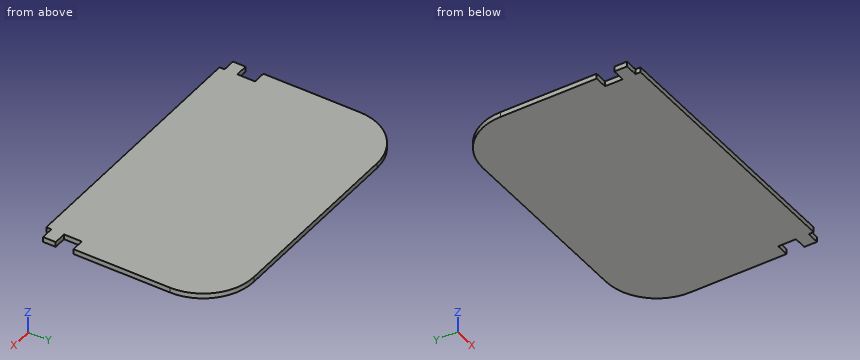
from build123d import *

# Parameters (mm, degrees)
BOSS_EXTRUDE1_DEPTH = 1


with BuildPart() as part:
    # Sketch1 → Boss-Extrude1 (new body)
    with BuildSketch(Plane.XY):
        with BuildLine():
            Line((0, 1), (2.5, 1))
            Line((2.5, 1), (2.5, 0))
            Line((2.5, 0), (54.5, 0))
            Line((54.5, 0), (54.5, 1))
            Line((54.5, 1), (57, 1))
            Line((57, 1), (57, 3.5))
            Line((57, 3.5), (54.5, 3.5))
            Line((54.5, 3.5), (54.5, 7))
            Line((54.5, 7), (57, 7))
            Line((57, 7), (57, 26))
            ThreePointArc((57, 26), (54.071067812, 33.071067812), (47, 36))
            Line((47, 36), (10, 36))
            ThreePointArc((10, 36), (2.928932188, 33.071067812), (0, 26))
            Line((0, 26), (0, 7))
            Line((0, 7), (2.5, 7))
            Line((2.5, 7), (2.5, 3.5))
            Line((2.5, 3.5), (0, 3.5))
            Line((0, 3.5), (0, 1))
        make_face()
    extrude(amount=BOSS_EXTRUDE1_DEPTH)


solid = part.part
The listing builds one solid part. Answer for the finished solid, in the listing's coordinates (mm). Give positions to 0.01 mm unless a question says otherwise; leave off trailing zeros. Loops run counter-clockwise (first coordinate to the right, second up) from the corner with the lowest first, then second, coordinate; pieces in that order, holes last.
Item 1: A cutting plane is placed at C-C (y = 34.5). Give the vertices of the cut face in (x, z).
Derived:
outline: (4.73, 0) - (52.27, 0) - (52.27, 1) - (4.73, 1) - close
Item 2: A cutting plane is placed at B-B (y = 5.5). Give the vertices of the cut face in (x, z), then the cut area to 3 significant figures.
Derived:
outline: (2.5, 0) - (54.5, 0) - (54.5, 1) - (2.5, 1) - close
area: 52.0 mm2
Item 3: Find the intervals of material crossed by line 1 along X through (y, z) = (26.5, 0.5); line 2 along Y through (x, z) = (4.5, 0.5); line 3 along Y through (x, z) = (3.5, 0.45), in increasing order.
Derived:
line 1: x = 0.01 to 56.99
line 2: y = 0 to 34.35
line 3: y = 0 to 33.6
Item 4: Each of these flat-tipped pins is pushed along its axis until it touches: pin 1 Ø0.5 at (x, z) = (1.5, 0.5) entering from -Y; pin 2 Ø0.5 at (y, z) = (0.5, 0.5) entering from +X. Where does it stop, or does it pass through?
Derived:
pin 1: stops at y = 1
pin 2: stops at x = 54.5
Item 5: A cutting plane is placed at A-A (z = 0.35). Give the vertices of the cut face in (x, y), then the cut area to 3 significant figures.
Derived:
outline: (0, 1) - (2.5, 1) - (2.5, 0) - (54.5, 0) - (54.5, 1) - (57, 1) - (57, 3.5) - (54.5, 3.5) - (54.5, 7) - (57, 7) - (57, 26) arc R10 ccw to (47, 36) - (10, 36) arc R10 ccw to (0, 26) - (0, 7) - (2.5, 7) - (2.5, 3.5) - (0, 3.5) - close
area: 1,990 mm2
